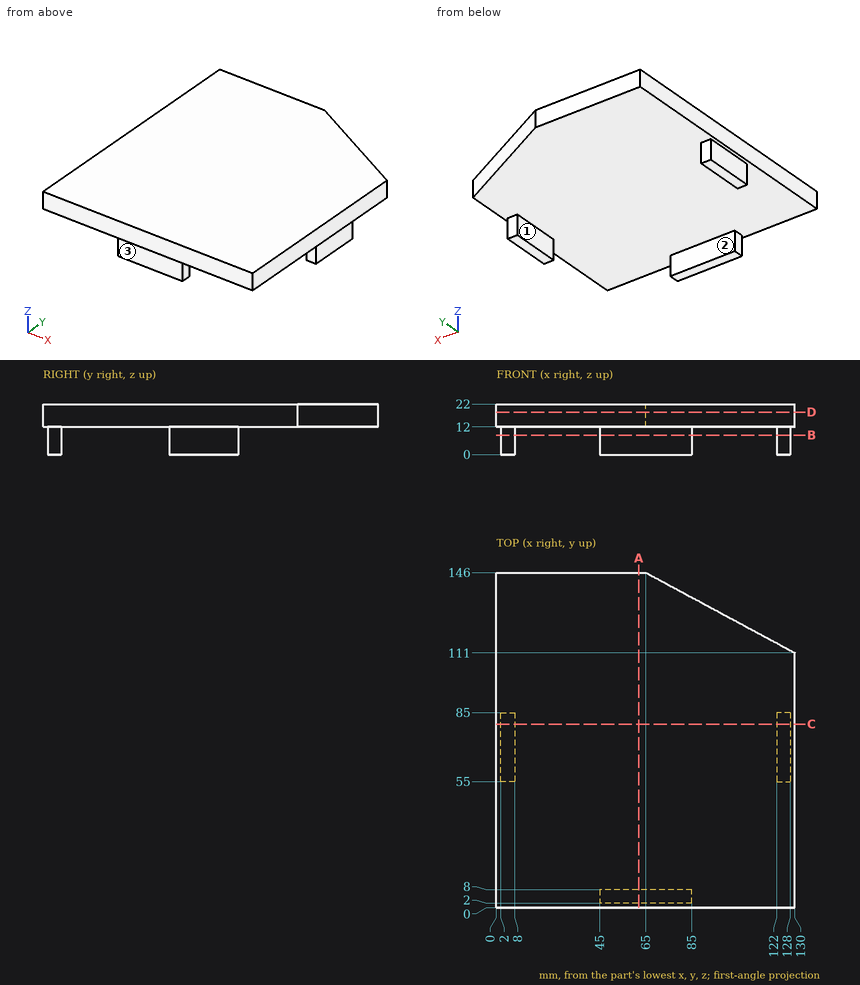
Here's the drawing with two shaded views (mm, measured from the low corner). I have some questions. A direction names the side the tool comes from. Coordinates: 2 decimals unless noted, no trailing zeros. Order: outer loops, then holes, each group sorted by start corner. A loop starts at its lowest first (then second) coordinate and runs counter-clockwise, first axis right, second up. Notation, with made-up numbers: M 4.25,-18 L 13.25,-18 A22 ccw 13.25,9 Z; hole C 69,89 d1. An arc over 180 degrees is marked long. Answer as CSV lines item,"result".
Item 1: Imagine slicing it at D-D on z = 18.5. Write out the boundary of the cut face in (x, y), plus the area to 3 significant figures.
Results found:
outline,"M 0,0 L 130,0 L 130,111 L 65,146 L 0,146 Z"
area,"17,800 mm2"
Item 2: If I drill on line 1 (X direction, y = 75.5, z = 9.5); line 2 (Z direction, x = 118, y = 110.5); line 3 (Y direction, x = 61.5, z = 2.75), over which ranges is the centre line in solid material (lowest first)?
Results found:
line 1,"2 to 8, 122 to 128"
line 2,"12 to 22"
line 3,"2 to 8"
Item 3: Imagine slicing it at B-B on z = 8.5. Write out the boundary of the cut face in (x, y), plus the area to 3 significant figures.
Results found:
outline,"M 2,55 L 8,55 L 8,85 L 2,85 Z; M 45,2 L 85,2 L 85,8 L 45,8 Z; M 122,55 L 128,55 L 128,85 L 122,85 Z"
area,"600 mm2"
Item 4: Imagine slicing it at A-A on x = 62. Write out the boundary of the cut face in (y, z), plus the area to 3 significant figures.
Results found:
outline,"M 0,12 L 2,12 L 2,0 L 8,0 L 8,12 L 146,12 L 146,22 L 0,22 Z"
area,"1,530 mm2"
Item 5: On a 3-axis mill with a long thin cutter (end or side, diameter ignored), from which of +Z, -Z, +X, -X, +Y, -Y can I reach the whole of each face in a straight line? I mean the marked faces 1, 2 and 3. Say none if no direction works.
Results found:
face 1,"-Z, +Y, -Y"
face 2,"-Z, +X, -X, +Y"
face 3,"-Z, +X, -X, -Y"
Item 6: For pin 1 (3.5 mm diameter, centred on x = 69, z = 3.5, fed in from -Y); pin 2 (6 mm diameter, centred on y = 73, z = 8, fed in from +X); pin 3 (5 mm diameter, centred on x = 4, z = 7, fed in from +Y); pin 4 (1 mm diameter, centred on y = 53.5, z = 4.5, fed in from +X), each with a flat end and sliding along its axis, tell me the tip position at first contact or that it passes through.
Results found:
pin 1,"y = 2"
pin 2,"x = 128"
pin 3,"y = 85"
pin 4,"through"
Item 7: Imagine slicing it at C-C on y = 80. Write out the boundary of the cut face in (x, z).
Results found:
outline,"M 0,12 L 2,12 L 2,0 L 8,0 L 8,12 L 122,12 L 122,0 L 128,0 L 128,12 L 130,12 L 130,22 L 0,22 Z"
